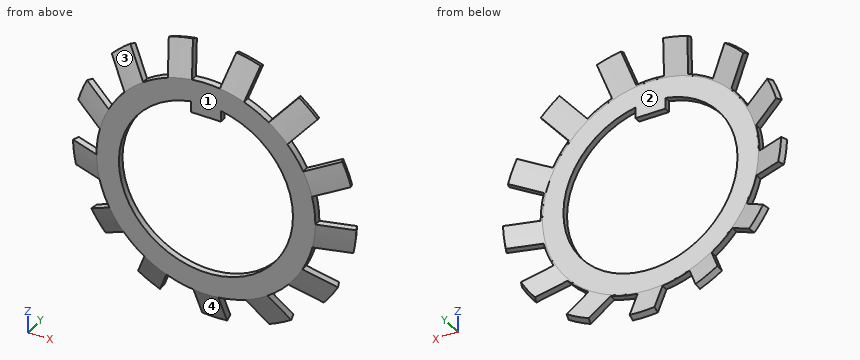
Solid Edge part; units mm, degrees
sketch "Sketch1" plane through (0, 0, 0) normal (1, 0, 0) x (0, 1, 0)
  line L0 (1.25, 0) -> (1.25, -21.7229)
  line L1 (1.25, -21.7229) -> (4.1639, -27.9717)
  line L2 (4.1639, -27.9717) -> (3.031, -28.5)
  line L3 (3.031, -28.5) -> (0, -22)
  line L4 (0, -22) -> (0, 0)
  line L5 (0, 0) -> (1.25, 0)
revolve "RevolvedProtrusion1" add sketch "Sketch1" angle 360 about axis through (0, -114, 0) along (0, 1, 0)
sketch "Sketch2" plane through (0, 0, 0) normal (0, -1, 0) x (1, 0, 0)
  arc A0 (3, 17.2409) -> (-3, 17.2409) centre (0, 0) cw
  line L0 (-3, 17.2409) -> (-3, 15)
  line L1 (-3, 15) -> (3, 15)
  line L2 (3, 15) -> (3, 17.2409)
extrude "Cutout1" cut sketch "Sketch2" against normal blind 114
sketch "Sketch3" plane through (0, 0, 0) normal (0, -1, 0) x (1, 0, 0)
  circle A0 centre (0, 0) radius 57
  line L0 (-28.4845, -0.9403) -> (-21.9995, -0.1529)
  arc A1 (-21.9995, -0.1529) -> (-21.3236, 5.4132) centre (0, 0) cw
  line L1 (-21.3236, 5.4132) -> (-27.4318, 7.7297)
  arc A2 (-27.4318, 7.7297) -> (-26.648, 10.1062) centre (0, 0) cw
  arc A3 (-26.648, 10.1062) -> (-25.6587, 12.4048) centre (0, 0) cw
  line L2 (-25.6587, 12.4048) -> (-19.5506, 10.0883)
  arc A4 (-19.5506, 10.0883) -> (-16.3655, 14.7028) centre (0, 0) cw
  line L3 (-16.3655, 14.7028) -> (-20.6974, 19.5925)
  arc A5 (-20.6974, 19.5925) -> (-18.899, 21.3326) centre (0, 0) cw
  arc A6 (-18.899, 21.3326) -> (-16.9549, 22.9081) centre (0, 0) cw
  line L4 (-16.9549, 22.9081) -> (-12.6229, 18.0184)
  arc A7 (-12.6229, 18.0184) -> (-7.6582, 20.6241) centre (0, 0) cw
  line L5 (-7.6582, 20.6241) -> (-9.2216, 26.9669)
  arc A8 (-9.2216, 26.9669) -> (-6.8205, 27.6718) centre (0, 0) cw
  arc A9 (-6.8205, 27.6718) -> (-4.3669, 28.1635) centre (0, 0) cw
  line L6 (-4.3669, 28.1635) -> (-2.8035, 21.8206)
  arc A10 (-2.8035, 21.8206) -> (2.8035, 21.8206) centre (0, 0) cw
  line L7 (2.8035, 21.8206) -> (4.3669, 28.1635)
  arc A11 (4.3669, 28.1635) -> (6.8205, 27.6718) centre (0, 0) cw
  arc A12 (6.8205, 27.6718) -> (9.2216, 26.9669) centre (0, 0) cw
  line L8 (9.2216, 26.9669) -> (7.6582, 20.6241)
  arc A13 (7.6582, 20.6241) -> (12.6229, 18.0184) centre (0, 0) cw
  line L9 (12.6229, 18.0184) -> (16.9549, 22.9081)
  arc A14 (16.9549, 22.9081) -> (18.899, 21.3326) centre (0, 0) cw
  arc A15 (18.899, 21.3326) -> (20.6974, 19.5925) centre (0, 0) cw
  line L10 (20.6974, 19.5925) -> (16.3655, 14.7028)
  arc A16 (16.3655, 14.7028) -> (19.5506, 10.0883) centre (0, 0) cw
  line L11 (19.5506, 10.0883) -> (25.6587, 12.4048)
  arc A17 (25.6587, 12.4048) -> (26.648, 10.1062) centre (0, 0) cw
  arc A18 (26.648, 10.1062) -> (27.4318, 7.7297) centre (0, 0) cw
  line L12 (27.4318, 7.7297) -> (21.3236, 5.4132)
  arc A19 (21.3236, 5.4132) -> (21.9995, -0.1529) centre (0, 0) cw
  line L13 (21.9995, -0.1529) -> (28.4845, -0.9403)
  arc A20 (28.4845, -0.9403) -> (28.2922, -3.4353) centre (0, 0) cw
  arc A21 (28.2922, -3.4353) -> (27.8818, -5.9038) centre (0, 0) cw
  line L14 (27.8818, -5.9038) -> (21.3968, -5.1164)
  arc A22 (21.3968, -5.1164) -> (19.4085, -10.359) centre (0, 0) cw
  line L15 (19.4085, -10.359) -> (24.7848, -14.07)
  arc A23 (24.7848, -14.07) -> (23.455, -16.1898) centre (0, 0) cw
  arc A24 (23.455, -16.1898) -> (21.9445, -18.1849) centre (0, 0) cw
  line L16 (21.9445, -18.1849) -> (16.5682, -14.4739)
  arc A25 (16.5682, -14.4739) -> (12.3713, -18.192) centre (0, 0) cw
  line L17 (12.3713, -18.192) -> (15.4072, -23.9764)
  arc A26 (15.4072, -23.9764) -> (13.2446, -25.2355) centre (0, 0) cw
  arc A27 (13.2446, -25.2355) -> (10.9799, -26.3) centre (0, 0) cw
  line L18 (10.9799, -26.3) -> (7.944, -20.5157)
  arc A28 (7.944, -20.5157) -> (2.5, -21.8575) centre (0, 0) cw
  line L19 (2.5, -21.8575) -> (2.5, -28.3901)
  arc A29 (2.5, -28.3901) -> (0, -28.5) centre (0, 0) cw
  arc A30 (0, -28.5) -> (-2.5, -28.3901) centre (0, 0) cw
  line L20 (-2.5, -28.3901) -> (-2.5, -21.8575)
  arc A31 (-2.5, -21.8575) -> (-7.944, -20.5157) centre (0, 0) cw
  line L21 (-7.944, -20.5157) -> (-10.9799, -26.3)
  arc A32 (-10.9799, -26.3) -> (-13.2446, -25.2355) centre (0, 0) cw
  arc A33 (-13.2446, -25.2355) -> (-15.4072, -23.9764) centre (0, 0) cw
  line L22 (-15.4072, -23.9764) -> (-12.3713, -18.192)
  arc A34 (-12.3713, -18.192) -> (-16.5682, -14.4739) centre (0, 0) cw
  line L23 (-16.5682, -14.4739) -> (-21.9445, -18.1849)
  arc A35 (-21.9445, -18.1849) -> (-23.455, -16.1898) centre (0, 0) cw
  arc A36 (-23.455, -16.1898) -> (-24.7848, -14.07) centre (0, 0) cw
  line L24 (-24.7848, -14.07) -> (-19.4085, -10.359)
  arc A37 (-19.4085, -10.359) -> (-21.3968, -5.1164) centre (0, 0) cw
  line L25 (-21.3968, -5.1164) -> (-27.8818, -5.9038)
  arc A38 (-27.8818, -5.9038) -> (-28.2922, -3.4353) centre (0, 0) cw
  arc A39 (-28.2922, -3.4353) -> (-28.4845, -0.9403) centre (0, 0) cw
extrude "ExtrudedCutout_2" cut sketch "Sketch3" against normal blind 114 and the other way blind 114
properties part number "sicherungsbl_din5406_65365301"
The listing builds one solid part. Answer for the finished solid, in the listing's coordinates (mm). Face numbers are marked on the shaded views. Coordinates: 2 decimals unless noted, no trailing zeros. Write each loop counter-clockwise with the first axis right and the second up, starting at its lowest first coordinate (ties: lowest second). Pieces come first, ordered by that corner, then holes. Notation, with made-up numbers: (78.25, 10.5) - (134.25, 10.5) arc R12 cw to (134.25, 31.5) - close; hole circle Ø1 at (15.5, -20.75). An arc over 180 degrees is marked (long way). Return JSON: item names as keys, results as strings. Group by question number.
1. Given pin 1 (1.4 mm diameter, centred on y = 1, z = 16.5, fed in from +X); pin 2 (5 mm diameter, centred on x = -16.5, z = -13, fed in from +Y); pin 3 (21 mm diameter, centred on x = 0, z = 0, fed in from +Y); pin 4 (1.4 mm diameter, centred on y = 1, z = 16, fed in from -X), each flat-ended and moving along its own axis, determine where each tip first touches the part or whether it passes through.
2. Straight lines are drawn through the part: L1, parallel to Z at x = 0, y = 0.7; L2, parallel to X at y = 0.9, z = 0; L3, parallel to X at y = 1.4, z = -5. For each, find the intervals that lie inside material, in ascending order.
3. Determine the mould class of the marked faces 1, 2, 3 and 4 for opening direction Z: released by +Z, released by -Z, zero draft, split by the parting line, or undercut.
4. A cutting plane is placed at B-B, the plane x = 14. Give the number of separate pieces and of enclosed holes in the cut face, plus the area to 3 significant figures.
5. A cutting plane is placed at A-A, the plane x = 0. Determine the outline of the cut face in (y, z).
Ans:
{
 "1": {"pin 1": "x = 18.43", "pin 2": "y = 2.08", "pin 3": "through", "pin 4": "x = -18.1"},
 "2": {"L1": "-23.5 to -17.5, 15 to 22", "L2": "-22 to -17.5, 17.5 to 22", "L3": "-24.5 to -21.47, 21.47 to 24.5"},
 "3": {"face 1": "zero draft", "face 2": "undercut", "face 3": "released by +Z", "face 4": "released by -Z"},
 "4": {"separate pieces": "3", "enclosed holes": "0", "area": "24.3 mm²"},
 "5": {"outline": "(0, -22) - (3.03, -28.5) - (4.16, -27.97) - (1.25, -21.72) - (1.25, -17.5) - (0, -17.5) - close; (0, 15) - (1.25, 15) - (1.25, 21.72) - (1.38, 22) - (0, 22) - close"}
}
